Model file for the job. Use its own axes, mm. Face numbers are marked on the shaded views. A direction names the side the tool comes from. Coordinates: 2 decimals unless noted, no trailing zeros. Loops run counter-clockwise (first coordinate to the right, second up) from the corner with the lowest first, then second, coordinate; pieces in that order, holes last. Notation, with made-up numbers: M -1,54 L 33,54 A20 ccw 33,91 Z; hole C -12.5,34.25 d10. An arc over 180 degrees is marked long. One line per question, with ' | ' between items. Start each with the question number.
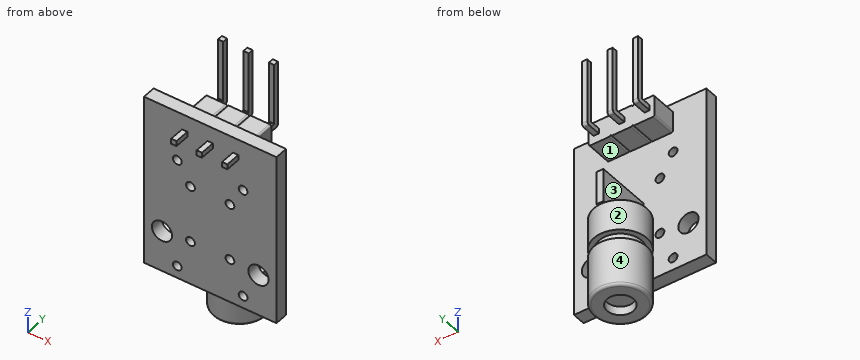
```python
from build123d import *

# Parameters (mm, degrees)
SKETCH1_W           = 15.1
SKETCH1_H           = 19.6
BOSS_EXTRUDE1_DEPTH = 1.5
SKETCH2_W           = 0.6
SKETCH2_H           = 0.6
BOSS_EXTRUDE2_DEPTH = 1.7
BOSS_EXTRUDE3_DEPTH = 2.9
SKETCH4_W           = 0.6
SKETCH4_H           = 0.6
BOSS_EXTRUDE4_DEPTH = 1.8
SKETCH5_W           = 0.6
SKETCH5_H           = 0.6
BOSS_EXTRUDE5_DEPTH = 7
SKETCH7_W           = 0.8
SKETCH7_H           = 3.8
BOSS_EXTRUDE6_DEPTH = 6.3
SKETCH8_R           = 3
BOSS_EXTRUDE7_DEPTH = 3.5
SKETCH9_R           = 2.4
BOSS_EXTRUDE8_DEPTH = 1
SKETCH10_R          = 3
BOSS_EXTRUDE9_DEPTH = 5.5
FILLET1_R           = 0.3
SKETCH11_R          = 1.5
CUT_EXTRUDE1_DEPTH  = 1
SKETCH12_R          = 1.15
CUT_EXTRUDE2_DEPTH  = 4.2
CUT_EXTRUDE3_REACH  = 9.8
SKETCH13_R          = 0.5
CUT_EXTRUDE4_REACH  = 9.8
SKETCH14_R          = 0.5
FILLET2_R           = 0.2
FILLET3_R           = 0.05
FILLET5_R           = 0.3


with BuildPart() as part:
    # Sketch1 → Boss-Extrude1 (new body)
    with BuildSketch(Plane(origin=(0, 0, 0), x_dir=(1, 0, 0), z_dir=(0, 1, 0))):
        Rectangle(SKETCH1_W, SKETCH1_H)
    extrude(amount=BOSS_EXTRUDE1_DEPTH)

    # Sketch2 → Boss-Extrude2 (add)
    with BuildSketch(Plane.XZ):
        with Locations((0, 7.7)):
            Rectangle(SKETCH2_W, SKETCH2_H)
        with Locations((2.9, 7.7)):
            Rectangle(SKETCH2_W, SKETCH2_H)
        with Locations((-2.9, 7.7)):
            Rectangle(SKETCH2_W, SKETCH2_H)
    extrude(amount=BOSS_EXTRUDE2_DEPTH)

    # Sketch3 → Boss-Extrude3 (add)
    with BuildSketch(Plane(origin=(0, 1.5, 0), x_dir=(1, 0, 0), z_dir=(0, 1, 0))):
        with BuildLine():
            Line((-3.75, -8.95), (-3.75, -6.45))
            Line((-3.75, -6.45), (-1.45, -6.45))
            ThreePointArc((-1.45, -6.45), (-1.308578644, -6.508578644), (-1.25, -6.65))
            ThreePointArc((-1.25, -6.65), (-1.191421356, -6.508578644), (-1.05, -6.45))
            Line((-1.05, -6.45), (1.05, -6.45))
            ThreePointArc((1.05, -6.45), (1.191421356, -6.508578644), (1.25, -6.65))
            ThreePointArc((1.25, -6.65), (1.308578644, -6.508578644), (1.45, -6.45))
            Line((1.45, -6.45), (3.75, -6.45))
            Line((3.75, -6.45), (3.75, -8.95))
            Line((3.75, -8.95), (1.45, -8.95))
            ThreePointArc((1.45, -8.95), (1.308578644, -8.891421356), (1.25, -8.75))
            ThreePointArc((1.25, -8.75), (1.191421356, -8.891421356), (1.05, -8.95))
            Line((1.05, -8.95), (-1.05, -8.95))
            ThreePointArc((-1.05, -8.95), (-1.191421356, -8.891421356), (-1.25, -8.75))
            ThreePointArc((-1.25, -8.75), (-1.308578644, -8.891421356), (-1.45, -8.95))
            Line((-1.45, -8.95), (-3.75, -8.95))
        make_face()
    extrude(amount=BOSS_EXTRUDE3_DEPTH)

    # Sketch4 → Boss-Extrude4 (add)
    with BuildSketch(Plane(origin=(0, 4.4, 0), x_dir=(1, 0, 0), z_dir=(0, 1, 0))):
        with Locations((-2.9, -7.7)):
            Rectangle(SKETCH4_W, SKETCH4_H)
        with Locations((0, -7.7)):
            Rectangle(SKETCH4_W, SKETCH4_H)
        with Locations((2.9, -7.7)):
            Rectangle(SKETCH4_W, SKETCH4_H)
    extrude(amount=BOSS_EXTRUDE4_DEPTH)

    # Sketch5 → Boss-Extrude5 (add)
    with BuildSketch(Plane.XY.offset(8)):
        with Locations((-2.9, 5.9)):
            Rectangle(SKETCH5_W, SKETCH5_H)
        with Locations((0, 5.9)):
            Rectangle(SKETCH5_W, SKETCH5_H)
        with Locations((2.9, 5.9)):
            Rectangle(SKETCH5_W, SKETCH5_H)
    extrude(amount=BOSS_EXTRUDE5_DEPTH)

    # Sketch7 → Boss-Extrude6 (add)
    with BuildSketch(Plane(origin=(0, 1.5, 0), x_dir=(1, 0, 0), z_dir=(0, 1, 0))):
        with Locations((0, 2.3)):
            Rectangle(SKETCH7_W, SKETCH7_H)
    extrude(amount=BOSS_EXTRUDE6_DEPTH)

    # Sketch8 → Boss-Extrude7 (add)
    with BuildSketch(Plane(origin=(0, 0, -4.2), x_dir=(-1, 0, 0), z_dir=(0, 0, -1))):
        with Locations((0, 4.6)):
            Circle(SKETCH8_R)
    extrude(amount=BOSS_EXTRUDE7_DEPTH)

    # Sketch9 → Boss-Extrude8 (add)
    with BuildSketch(Plane(origin=(0, 0, -7.7), x_dir=(-1, 0, 0), z_dir=(0, 0, -1))):
        with Locations((0, 4.6)):
            Circle(SKETCH9_R)
    extrude(amount=BOSS_EXTRUDE8_DEPTH)

    # Sketch10 → Boss-Extrude9 (add)
    with BuildSketch(Plane(origin=(0, 0, -8.7), x_dir=(-1, 0, 0), z_dir=(0, 0, -1))):
        with Locations((0, 4.6)):
            Circle(SKETCH10_R)
    extrude(amount=BOSS_EXTRUDE9_DEPTH)

    # Fillet1
    fillet1_edges = [part.edges().sort_by_distance(p)[0] for p in [
        (3, 4.6, -14.2),
    ]]
    fillet(fillet1_edges, radius=FILLET1_R)

    # Sketch11 → Cut-Extrude1 (cut)
    with BuildSketch(Plane(origin=(0, 0, -14.2), x_dir=(-1, 0, 0), z_dir=(0, 0, -1))):
        with Locations((0, 4.6)):
            Circle(SKETCH11_R)
    extrude(amount=-CUT_EXTRUDE1_DEPTH, mode=Mode.SUBTRACT)

    # Sketch12 → Cut-Extrude2 (cut, through all)
    with BuildSketch(Plane(origin=(0, 1.5, 0), x_dir=(1, 0, 0), z_dir=(0, 1, 0))):
        with Locations((-5.5, 5.1)):
            Circle(SKETCH12_R)
        with Locations((5.5, 5.1)):
            Circle(SKETCH12_R)
    extrude(amount=-CUT_EXTRUDE2_DEPTH, mode=Mode.SUBTRACT)

    # Sketch13 → Cut-Extrude3 (cut, up to next)
    with BuildSketch(Plane.XZ, mode=Mode.PRIVATE) as cut_extrude3_sk1:
        with Locations((-2.25, -4.8)):
            Circle(SKETCH13_R)
    cut_extrude3_tool1 = extrude(cut_extrude3_sk1.sketch, amount=-CUT_EXTRUDE3_REACH, mode=Mode.PRIVATE) & part.part
    add(cut_extrude3_tool1.solids().sort_by_distance((-2.25, 0, -4.8))[0], mode=Mode.SUBTRACT)
    # Sketch13 → Cut-Extrude3 (cut, up to next)
    with BuildSketch(Plane.XZ, mode=Mode.PRIVATE) as cut_extrude3_sk2:
        with Locations((2.25, -4.8)):
            Circle(SKETCH13_R)
    cut_extrude3_tool2 = extrude(cut_extrude3_sk2.sketch, amount=-CUT_EXTRUDE3_REACH, mode=Mode.PRIVATE) & part.part
    add(cut_extrude3_tool2.solids().sort_by_distance((2.25, 0, -4.8))[0], mode=Mode.SUBTRACT)
    # Sketch13 → Cut-Extrude3 (cut, up to next)
    with BuildSketch(Plane.XZ, mode=Mode.PRIVATE) as cut_extrude3_sk3:
        with Locations((2.25, 1.7)):
            Circle(SKETCH13_R)
    cut_extrude3_tool3 = extrude(cut_extrude3_sk3.sketch, amount=-CUT_EXTRUDE3_REACH, mode=Mode.PRIVATE) & part.part
    add(cut_extrude3_tool3.solids().sort_by_distance((2.25, 0, 1.7))[0], mode=Mode.SUBTRACT)
    # Sketch13 → Cut-Extrude3 (cut, up to next)
    with BuildSketch(Plane.XZ, mode=Mode.PRIVATE) as cut_extrude3_sk4:
        with Locations((-2.25, 1.7)):
            Circle(SKETCH13_R)
    cut_extrude3_tool4 = extrude(cut_extrude3_sk4.sketch, amount=-CUT_EXTRUDE3_REACH, mode=Mode.PRIVATE) & part.part
    add(cut_extrude3_tool4.solids().sort_by_distance((-2.25, 0, 1.7))[0], mode=Mode.SUBTRACT)

    # Sketch14 → Cut-Extrude4 (cut, up to next)
    with BuildSketch(Plane.XZ, mode=Mode.PRIVATE) as cut_extrude4_sk1:
        with Locations((3.75, 4.1)):
            Circle(SKETCH14_R)
    cut_extrude4_tool1 = extrude(cut_extrude4_sk1.sketch, amount=-CUT_EXTRUDE4_REACH, mode=Mode.PRIVATE) & part.part
    add(cut_extrude4_tool1.solids().sort_by_distance((3.75, 0, 4.1))[0], mode=Mode.SUBTRACT)
    # Sketch14 → Cut-Extrude4 (cut, up to next)
    with BuildSketch(Plane.XZ, mode=Mode.PRIVATE) as cut_extrude4_sk2:
        with Locations((-3.75, 4.1)):
            Circle(SKETCH14_R)
    cut_extrude4_tool2 = extrude(cut_extrude4_sk2.sketch, amount=-CUT_EXTRUDE4_REACH, mode=Mode.PRIVATE) & part.part
    add(cut_extrude4_tool2.solids().sort_by_distance((-3.75, 0, 4.1))[0], mode=Mode.SUBTRACT)
    # Sketch14 → Cut-Extrude4 (cut, up to next)
    with BuildSketch(Plane.XZ, mode=Mode.PRIVATE) as cut_extrude4_sk3:
        with Locations((-3.75, -8.4)):
            Circle(SKETCH14_R)
    cut_extrude4_tool3 = extrude(cut_extrude4_sk3.sketch, amount=-CUT_EXTRUDE4_REACH, mode=Mode.PRIVATE) & part.part
    add(cut_extrude4_tool3.solids().sort_by_distance((-3.75, 0, -8.4))[0], mode=Mode.SUBTRACT)
    # Sketch14 → Cut-Extrude4 (cut, up to next)
    with BuildSketch(Plane.XZ, mode=Mode.PRIVATE) as cut_extrude4_sk4:
        with Locations((3.75, -8.4)):
            Circle(SKETCH14_R)
    cut_extrude4_tool4 = extrude(cut_extrude4_sk4.sketch, amount=-CUT_EXTRUDE4_REACH, mode=Mode.PRIVATE) & part.part
    add(cut_extrude4_tool4.solids().sort_by_distance((3.75, 0, -8.4))[0], mode=Mode.SUBTRACT)

    # Fillet2
    fillet2_edges = [part.edges().sort_by_distance(p)[0] for p in [
        (-3.75, 2.95, 8.95),
        (3.75, 2.95, 8.95),
        (3.75, 2.95, 6.45),
        (-3.75, 2.95, 6.45),
    ]]
    fillet(fillet2_edges, radius=FILLET2_R)

    # Fillet3
    fillet3_edges = [part.edges().sort_by_distance(p)[0] for p in [
        (-2.9, 5.6, 8),
        (0, 5.6, 8),
        (2.9, 5.6, 8),
    ]]
    fillet(fillet3_edges, radius=FILLET3_R)

    # Fillet5
    fillet5_edges = [part.edges().sort_by_distance(p)[0] for p in [
        (0, 6.2, 7.4),
        (2.9, 6.2, 7.4),
        (-2.9, 6.2, 7.4),
    ]]
    fillet(fillet5_edges, radius=FILLET5_R)


solid = part.part
```
(1) Band-saw the part on A-A on x = 5.5. Write the cut outline in (y, z), then the cut area to 4 significant figures.
(2) Band-saw the part on B-B on z = -9.25. Write the cut outline in (x, y).
(3) 3-axis set-ups, long thin cutter, end or side, ignore diameter. For the marked faces 1 and 2: which of +Z, -Z, +X, -X, +Y, -Y reach the whole face in a straight line?
(4) Band-saw the part on D-D on y = 0.5. Give the number of separate pieces and of enclosed holes in the cut face, then the cut area to 3 significant figures.
(5) Two-plate mould, pull along Z, no slides. Class the marked faces 3 and 4: pulls with the +Z half, pulls with the -Z half, needs draft (parallel to the pull), parting line crosses it, or undercut.
(6) Pin check, flat tips, straight feed: P1, Ø2, axis at y = 4.5, z = -7, coming from the -X side; P2, Ø2.5, axis at x = 0.5, y = 3.5, coming from the +Z side; P3, Ø0.9, axis at y = 5.5, z = 9.5, coming from the +X side; P4, Ø3, axis at x = -5.5, y = 6.5, coming from the -Z side. Stop position of each tip, or through.
(7) Drill centre lines: line 1 (Z direction, x = 2.25, y = 0.6); line 2 (Z direction, x = -3.75, y = 0.3); line 3 (Z direction, x = 5.5, y = 0.95). Where is each one in solid material? Low to high. Write a range as [from, to].
(8) Band-saw the part on C-C on z = 1.7. Write the cut outline in (x, y).
Computed values:
1) outline: M 0,-9.8 L 1.5,-9.8 L 1.5,-6.25 L 0,-6.25 Z; M 0,-3.95 L 1.5,-3.95 L 1.5,9.8 L 0,9.8 Z | area: 25.95 mm^2
2) outline: M -7.55,0 L 7.55,0 L 7.55,1.5 L -7.55,1.5 Z; C 0,4.6 d6
3) face 1: +X, -X, +Y | face 2: -Z
4) separate pieces: 1 | enclosed holes: 10 | area: 281 mm^2
5) face 3: undercut | face 4: needs draft
6) P1: x = -3 | P2: z = 8.95 | P3: x = 3.2 | P4: through
7) line 1: [-9.8, -5.3], [-4.3, 1.2], [2.2, 9.8] | line 2: [-9.8, -8.9], [-7.9, 3.6], [4.6, 9.8] | line 3: [-9.8, -6.25], [-3.95, 9.8]
8) outline: M -7.55,0 L -2.75,0 L -2.75,1.5 L -7.55,1.5 Z; M -1.75,0 L 1.75,0 L 1.75,1.5 L -1.75,1.5 Z; M 2.75,0 L 7.55,0 L 7.55,1.5 L 2.75,1.5 Z
